Autodesk Inventor part; units mm, degrees
ref_plane "YZ Plane" through (0, 0, 0) normal (1, 0, 0) x (0, 1, 0)
ref_plane "XZ Plane" through (0, 0, 0) normal (0, 1, 0) x (-1, 0, 0)
ref_plane "XY Plane" through (0, 0, 0) normal (0, 0, 1) x (1, 0, 0)
sketch "Sketch1" plane through (0, 0, 0) normal (0, 0, 1) x (1, 0, 0)
  circle A0 centre (0, 0) radius 7.5
  dimension "d0" = 15
extrude "Extrusion1" add sketch "Sketch1" along normal blind 10
sketch "Sketch2" plane through (0, 0, 0) normal (0, 0, -1) x (-1, 0, 0)
  line L0 (-20, -20) -> (20, -20)
  line L1 (20, -20) -> (20, 20)
  line L2 (20, 20) -> (-20, 20)
  line L3 (-20, 20) -> (-20, -20)
  line L4 (-20, -20) -> (20, 20) construction
  line L5 (20, -20) -> (-20, 20) construction
  point P0 (0, 0)
  dimension "d3" = 40
  dimension "d4" = 40
extrude "Extrusion2" add sketch "Sketch2" along normal blind 30
fillet "Fillet1" radius 10 4 edges at (-20, 20, -15) (-20, -20, -15) (20, -20, -15) (20, 20, -15)
equation "\"d4\" = d3"
properties part number "MotorEslabon" material "Steel"
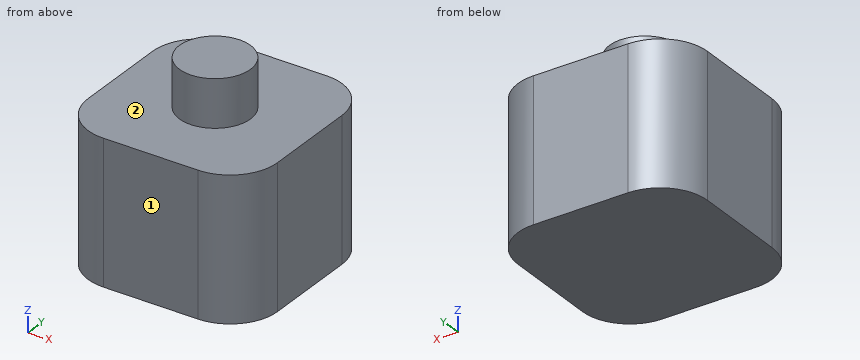
The listing builds one solid part. Answer for the finished solid, in the listing's coordinates (mm). Face numbers are marked on the shaded views. A direction names the side the tool comes from. Round coordinates to 2 decimals unless told otherwise and drop trailing zeros. Loops run counter-clockwise (first coordinate to the right, second up) from the corner with the lowest first, then second, coordinate; pieces in that order, holes last. Notation, with made-up numbers: M 71.25,44.5 L 82.25,44.5 A30 ccw 82.25,73.5 Z; hole C -5,51.5 d4. An arc over 180 degrees is marked long. Write each question's results on one line, items separated by ' | '. Start each with the question number.
1) Find section C-C on x = 15.5. Write down the section's boundary in (y, z), plus the area to 3 significant figures.
2) Find section D-D on z = 4.5. Write down the section's boundary in (x, y).
3) Straight lines are drawn through the part: probe 1 along Z at (x, y) = (-8, 14.5); probe 2 along Y at (x, z) = (-12, -26.5); probe 3 along X at (y, z) = (-13, -4). For each, find the intervals that lie inside material, in ascending order.
4) This flat-tipped pin is pushed along its axis until it touches: pin 1 (2 mm diameter, centred on x = -15, y = -14, fed in from +Z). Where does it stop, or does it pass through?
5) Which of the six approach directions +Z, -Z, +X, -X, +Y, -Y give full straight-line access (tool end or side, diameter ignored) to the marked faces 1 and 2?
6) Find section B-B on z = -18. Write down the section's boundary in (x, y).
7) Find section A-A on y = 0. Write down the section's boundary in (x, z), plus the area to 3 significant figures.
Final values:
1) outline: M -18.35,-30 L 18.35,-30 L 18.35,0 L -18.35,0 Z | area: 1,100 mm²
2) outline: C 0,0 d15
3) probe 1: -30 to 0 | probe 2: -19.8 to 19.8 | probe 3: -19.54 to 19.54
4) pin 1: z = 0
5) face 1: +Z, -Z, +X, -X, -Y | face 2: +Z
6) outline: M -20,-10 A10 ccw -10,-20 L 10,-20 A10 ccw 20,-10 L 20,10 A10 ccw 10,20 L -10,20 A10 ccw -20,10 Z
7) outline: M -20,-30 L 20,-30 L 20,0 L 7.5,0 L 7.5,10 L -7.5,10 L -7.5,0 L -20,0 Z | area: 1,350 mm²
